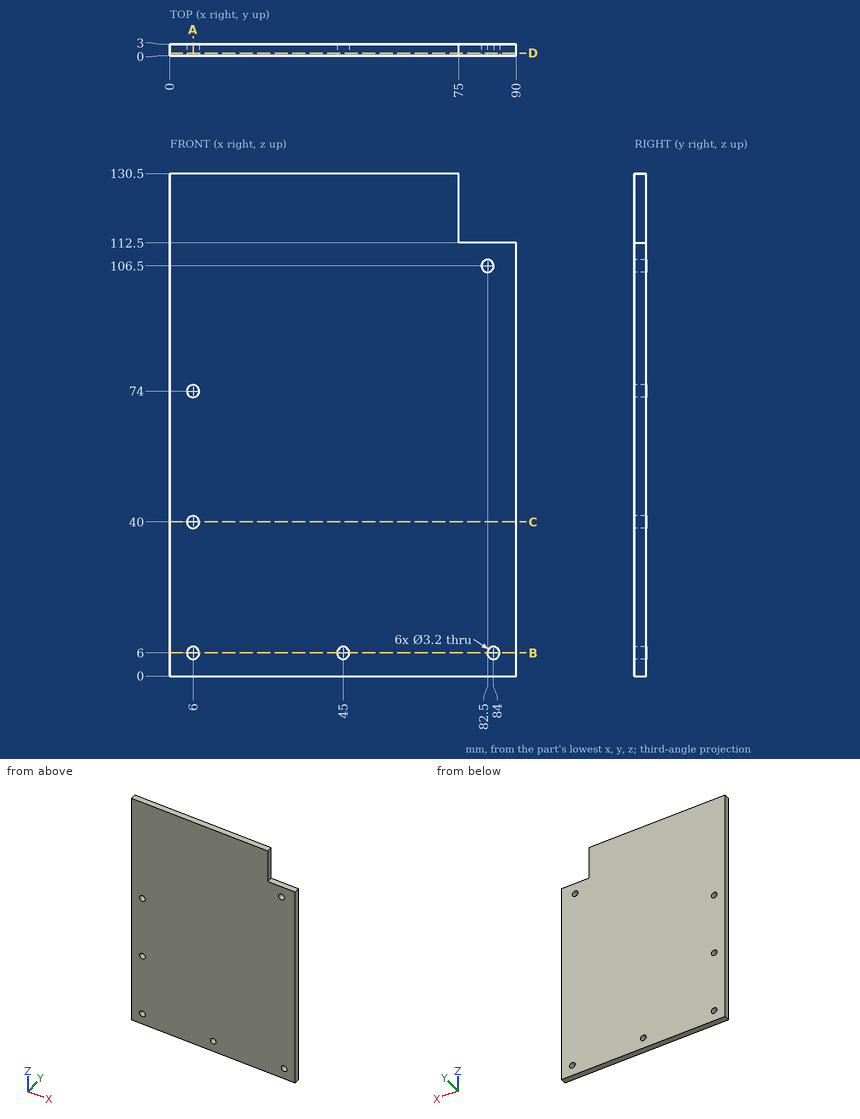
The drawing under review shows one solid part. Ordinate dimensions are in mm from its lowest x, y, z. Round coordinates to 2 decimals unless told otherwise and drop trailing zeros. Loops run counter-clockwise (first coordinate to the right, second up) from the corner with the lowest first, then second, coordinate; pieces in that order, holes last. Notation, with made-up numbers: (77.5, 12.25) - (129.5, 12.25) arc R29 ccw to (129.5, 45.25) - close; hole circle Ø8 at (68.5, -17). An arc over 180 degrees is marked (long way). One line per item, written item: value. Start each with the question number.
1) Consider section C-C on z = 40. Give the boundary of the cut face in (x, y).
2) Consider section B-B on z = 6. Give the boundary of the cut face in (x, y), then the cut area to 3 significant figures.
3) Consider section A-A on x = 6. Give the boundary of the cut face in (y, z), then the cut area to 3 significant figures.
4) Insertion check: pin 1 Ø3 at (x, z) = (6, 40) entering from -Y. The pin has a flat end and moves straight along its axis. Give the tip position at first contact, or say it passes through.
5) To check wall thickness, follow L1, parallel to X at y = 1.4, z = 6; L2, parallel to Z at x = 6, y = 1.9; L3, parallel to Z at x = 44.5, y = 2.9. State the ranges of each line that lie inside material, in increasing order. Write a range as from..to.
6) Consider section D-D on y = 0.65. Give the boundary of the cut face in (x, z), then the cut area to 3 significant figures.
Reported:
1. outline: (0, 0) - (4.4, 0) - (4.4, 3) - (0, 3) - close; (7.6, 0) - (90, 0) - (90, 3) - (7.6, 3) - close
2. outline: (0, 0) - (4.4, 0) - (4.4, 3) - (0, 3) - close; (7.6, 0) - (43.4, 0) - (43.4, 3) - (7.6, 3) - close; (46.6, 0) - (82.4, 0) - (82.4, 3) - (46.6, 3) - close; (85.6, 0) - (90, 0) - (90, 3) - (85.6, 3) - close
2. area: 241 mm^2
3. outline: (0, 0) - (3, 0) - (3, 4.4) - (0, 4.4) - close; (0, 7.6) - (3, 7.6) - (3, 38.4) - (0, 38.4) - close; (0, 41.6) - (3, 41.6) - (3, 72.4) - (0, 72.4) - close; (0, 75.6) - (3, 75.6) - (3, 130.5) - (0, 130.5) - close
3. area: 363 mm^2
4. pin 1: passes through
5. L1: x = 0..4.4, 7.6..43.4, 46.6..82.4, 85.6..90
5. L2: z = 0..4.4, 7.6..38.4, 41.6..72.4, 75.6..130.5
5. L3: z = 0..4.48, 7.52..130.5
6. outline: (0, 0) - (90, 0) - (90, 112.5) - (75, 112.5) - (75, 130.5) - (0, 130.5) - close; hole circle Ø3.2 at (6, 6); hole circle Ø3.2 at (6, 40); hole circle Ø3.2 at (6, 74); hole circle Ø3.2 at (45, 6); hole circle Ø3.2 at (82.5, 106.5); hole circle Ø3.2 at (84, 6)
6. area: 11,400 mm^2
